from build123d import *

# Parameters (mm, degrees)
ESQUISSE1_R             = 1.5
BOSS_EXTRU_1_DEPTH      = 5
BOSS_EXTRU_2_DEPTH      = 5
ESQUISSE4_W             = 5
ESQUISSE4_H             = 15
ENL_V_MAT_EXTRU_1_DEPTH = 10


with BuildPart() as part:
    # Esquisse1 → Boss.-Extru.1 (new body)
    with BuildSketch(Plane.XY):
        Polygon((0, 0), (32, 0), (32, -5), (37, -5), (37, 0), (37, 18), (22, 18), (12, 47), (0, 47), align=None)
        with Locations((6, 32)):
            Circle(ESQUISSE1_R, mode=Mode.SUBTRACT)
        with Locations((31, 12)):
            Circle(ESQUISSE1_R, mode=Mode.SUBTRACT)
    extrude(amount=BOSS_EXTRU_1_DEPTH)

    # Esquisse2 → Boss.-Extru.2 (add)
    with BuildSketch(Plane(origin=(0, 0, 0), x_dir=(-1, 0, 0), z_dir=(0, 0, -1))):
        with BuildLine():
            Line((-37, 0), (-65, 0))
            Line((-65, 0), (-65, -5))
            Line((-65, -5), (-70, -5))
            Line((-70, -5), (-70, 0))
            Line((-70, 0), (-75.5, 0))
            add(Edge.make_bspline(
                [(-75.5, 0), (-75.5, 5.982232529), (-67.685409636, 18), (-37, 18)],
                knots=[0, 0, 0, 0, 1, 1, 1, 1], degree=3))
            Line((-37, 18), (-37, 0))
        make_face()
        Polygon((42, 0), (47.5, 0), (47.5, 20), (65.5, 20), (65.5, 30), (47.5, 30), (47.5, 50), (65.5, 50), (65.5, 60), (47.5, 60), (47.5, 70), (20, 70), (20, 55), (0, 55), (0, 15), (42, 15), align=None)
        Polygon((-30, 18), (-22, 18), (-20.620689655, 22), (-30, 22), align=None)
    extrude(amount=-BOSS_EXTRU_2_DEPTH)

    # Esquisse4 → Enlèv. mat.-Extru.1 (cut)
    with BuildSketch(Plane(origin=(0, 0, 0), x_dir=(-1, 0, 0), z_dir=(0, 0, -1))):
        with Locations((-2.5, 7.5)):
            Rectangle(ESQUISSE4_W, ESQUISSE4_H)
    extrude(amount=-ENL_V_MAT_EXTRU_1_DEPTH, mode=Mode.SUBTRACT)


solid = part.part
Input: part model. Units: mm. Frame: model coordinates. A direction names the side the tool comes from. Round coordinates to 2 decimals unless told otherwise and drop trailing zeros. Order: outer loops, then holes, each group sorted by start corner. A loop starts at its lowest first (then second) coordinate and runs counter-clockwise, first axis right, second up. Notation, with made-up numbers: (63, -5) - (121, -5) arc R19 cw to (121, 27) - close; hole circle Ø6 at (13.5, 6). An arc over 180 degrees is marked (long way). Answer as a JSON object with one key per item and string values. Group by question number.
(1) Draft query along Y for faces 6 (the face through (-12, 33, 5)), 7 (the face through (67, -5, 2)), 8 (the face through (-56, 50, 2)). Return one class per face: released by +Y, released by -Y, zero draft, split by the parting line, or undercut.
(2) Reachability of faces 1 (the face through (-47.5, 40, 2)), 2 (the face through (70, -3, 2)), 3 (the face through (32, -2, 2)), 4 (the face through (-18, 15, 2)), 5 (the face through (-20, 63, 2)) from +Z, -Z, +X, -X, +Y, -Y: full face, straight path, thin tool, end or side. Return the list, or none.
(3) Cut plane B-B (z = 2.7). Count the separate pieces of the cut face and the enclosed holes in it, then the cut area to 3 significant figures.
(4) Pin query (flat end, axial travel): P1, Ø2, axis at x = 58, z = 3.5, coming from the +Y side; P2, Ø2.5, axis at x = -53.5, z = 1.5, coming from the +Y side; P3, Ø2.5, axis at y = -3, z = 3, coming from the -X side. Return the tip coordinate at first contact, or that it passes through.
(5) Cut plane A-A (y = 32). Return loops of the section in (x, z).
(6) Cut plane C-C (x = 19). Return loops of the section in (y, z).
(7) Material intervals for probe 1 along Y at (x, z) = (31, 1.8); probe 2 along X at (y, z) = (-1, 3.35); probe 3 along Y at (x, z) = (6, 1.15), sorted ascending. Write a range as from..to.
Here are the results:
{
 "1": {"face 6": "zero draft", "face 7": "released by -Y", "face 8": "undercut"},
 "2": {"face 1": "+Z, -Z, -X", "face 2": "+Z, -Z, +X, -Y", "face 3": "+Z, -Z, -X, -Y", "face 4": "+Z, -Z, -Y", "face 5": "+Z, -Z, +X, +Y"},
 "3": {"separate pieces": "1", "enclosed holes": "2", "area": "4,460 mm^2"},
 "4": {"P1": "stops at y = 15.77", "P2": "stops at y = 60", "P3": "stops at x = 32"},
 "5": {"outline": "(-47.5, 0) - (4.5, 0) - (4.5, 5) - (-47.5, 5) - close; (7.5, 0) - (17.17, 0) - (17.17, 5) - (7.5, 5) - close"},
 "6": {"outline": "(0, 0) - (26.7, 0) - (26.7, 5) - (0, 5) - close"},
 "7": {"probe 1": "y = 0..10.5, 13.5..18", "probe 2": "x = 32..37, 65..70", "probe 3": "y = 0..30.5, 33.5..47"}
}
